```python
from build123d import *

# Parameters (mm, degrees)
F0_W          = 153.443813324
F0_H          = 96.1026027799
F1_DEPTH      = 63.5
F2_R          = 11.6088535247
F2_R_2        = 12.4265954899
F3_DEPTH      = 25.4
F5_DEPTH      = 96.1036027799
F6_DEPTH      = 109.474
F6_DEPTH_BACK = 11.684


with BuildPart() as f1:
    # F0 (on Top) → F1 (new body)
    with BuildSketch(Plane.XY):
        Rectangle(F0_W, F0_H)
    extrude(amount=F1_DEPTH)

    # F2 (on face) → F3 (cut)
    with BuildSketch(Plane.XY.offset(63.5)):
        with Locations((-47.329030931, 0)):
            Circle(F2_R)
        with Locations((44.1418252885, 0)):
            Circle(F2_R_2)
    extrude(amount=-F3_DEPTH, mode=Mode.SUBTRACT)

    # F4 (on face) → F5 (cut, through all)
    with BuildSketch(Plane.XZ.offset(48.0513013899)):
        with BuildLine():
            ThreePointArc((-13.1851819962, 63.5), (0, 50.3148180038), (13.1851819962, 63.5))
            Line((13.1851819962, 63.5), (-13.1851819962, 63.5))
        make_face()
    extrude(amount=-F5_DEPTH, mode=Mode.SUBTRACT)

    # F4 (on face) → F6 (join, two sides)
    with BuildSketch(Plane.XZ.offset(48.0513013899)) as f6_sk:
        with BuildLine():
            ThreePointArc((-22.9800063856, 63.5), (0, 40.5199936144), (22.9800063856, 63.5))
            Line((22.9800063856, 63.5), (13.1851819962, 63.5))
            ThreePointArc((13.1851819962, 63.5), (0, 50.3148180038), (-13.1851819962, 63.5))
            Line((-13.1851819962, 63.5), (-22.9800063856, 63.5))
        make_face()
    extrude(amount=-F6_DEPTH)
    extrude(f6_sk.sketch, amount=F6_DEPTH_BACK)


solid = f1.part
```
The model under review builds one solid part; all positions refer to its coordinate system, in mm. A direction names the side the tool comes from. Round coordinates to 2 decimals unless told otherwise and drop trailing zeros. Loops run counter-clockwise (first coordinate to the right, second up) from the corner with the lowest first, then second, coordinate; pieces in that order, holes last. Notation, with made-up numbers: (-27, 29.5) - (-21, 29.5) arc R13 ccw to (-21, 53.5) - close; hole circle Ø7 at (87, -25.5). An arc over 180 degrees is marked (long way). Use a Markdown table: item, result. Add a question column.
Q1. Add section D-D (y = 19). State the section outline as (x, z) points, plus the area to 3 significant figures.
Q2. Add section B-B (x = 0). State the section outline as (y, z) points, plus the area to 3 significant figures.
Q3. Insertion check: pin 1 Ø10 at (x, z) = (-4.5, 32.5) entering from +Y; pin 2 Ø1.5 at (x, z) = (44, 23.5) entering from -Y; pin 3 Ø7.5 at (x, y) = (40, -4) entering from +Z. Each pin has a flat end and moves straight along its axis. Give the tip position at first contact, or say it passes through.
Q4. Machinability: for faces 4 (the face through (0.29, 1.69, 50.32)), 5 (the face through (-36.605, -4.446, 50.978)), 6 (the face through (-0.505, -53.812, 40.526)), 7 (the face through (-1, 48.051, 31)), which of the approach directions +Z, -Z, +X, -X, +Y, -Y give a long, thin tool a straight path to every point of the face, cutting with its end or side? Answer none if there is none.
Q5. For probe 1 along Z at (x, y) = (45.5, 4); probe 2 along Y at (x, z) = (41, 32); probe 3 along X at (y, z) = (14.5, 55.5), list the stretches that pass through material, from the lowest coordinate up.
Q6. Add section A-A (y = 0). State the section outline as (x, z) points.
Q7. The part is to be moulded in two halves that separate along X. For faces 1 (the face through (-47, 0, 38.1)), 2 (the face through (-76.722, -1, 31)), 3 (the face through (-1, -48.051, 31)), say which applies: pulls with the +X half, pulls with the -X half, needs draft (parallel to the pull), parting line crosses it, or undercut.
Q8. Add section C-C (z = 21). State the section outline as (x, y) points, plus the area to 3 significant figures.
Worked answers:
| question | item | result |
|---|---|---|
| 1 | outline | (-76.72, 0) - (76.72, 0) - (76.72, 63.5) - (13.19, 63.5) arc R13.19 cw to (-13.19, 63.5) - (-76.72, 63.5) - close |
| 1 | area | 9,470 mm² |
| 2 | outline | (-59.74, 40.52) - (-48.05, 40.52) - (-48.05, 0) - (48.05, 0) - (48.05, 40.52) - (61.42, 40.52) - (61.42, 50.31) - (-59.74, 50.31) - close |
| 2 | area | 5,080 mm² |
| 3 | pin 1 | y = 48.05 |
| 3 | pin 2 | y = -48.05 |
| 3 | pin 3 | z = 38.1 |
| 4 | face 4 | +Z, +Y, -Y |
| 4 | face 5 | +Z |
| 4 | face 6 | -Z, -Y |
| 4 | face 7 | -Z, +Y |
| 5 | probe 1 | 0 to 38.1 |
| 5 | probe 2 | -48.05 to 48.05 |
| 5 | probe 3 | -76.72 to -10.48, 10.48 to 76.72 |
| 6 | outline | (-76.72, 0) - (76.72, 0) - (76.72, 63.5) - (56.57, 63.5) - (56.57, 38.1) - (31.72, 38.1) - (31.72, 63.5) - (13.19, 63.5) arc R13.19 cw to (-13.19, 63.5) - (-35.72, 63.5) - (-35.72, 38.1) - (-58.94, 38.1) - (-58.94, 63.5) - (-76.72, 63.5) - close |
| 7 | face 1 | undercut |
| 7 | face 2 | pulls with the -X half |
| 7 | face 3 | needs draft |
| 8 | outline | (-76.72, -48.05) - (76.72, -48.05) - (76.72, 48.05) - (-76.72, 48.05) - close |
| 8 | area | 14,700 mm² |
